Geometry: see drawing. Coordinates: mm, zero at the bounding-box minimum. A direction names the side the tool comes from. Coordinates: 2 decimals unless noted, no trailing zeros. Loops run counter-clockwise (first coordinate to the right, second up) from the corner with the lowest first, then second, coordinate; pieces in that order, holes last. Notation, with made-up numbers: (36.25, -2) -> (76.25, -2) arc R18 cw to (76.25, 10) -> close; hole circle Ø4 at (33.25, 12.5). An arc over 180 degrees is marked (long way). One line per item, written item: value. Start each with the question number.
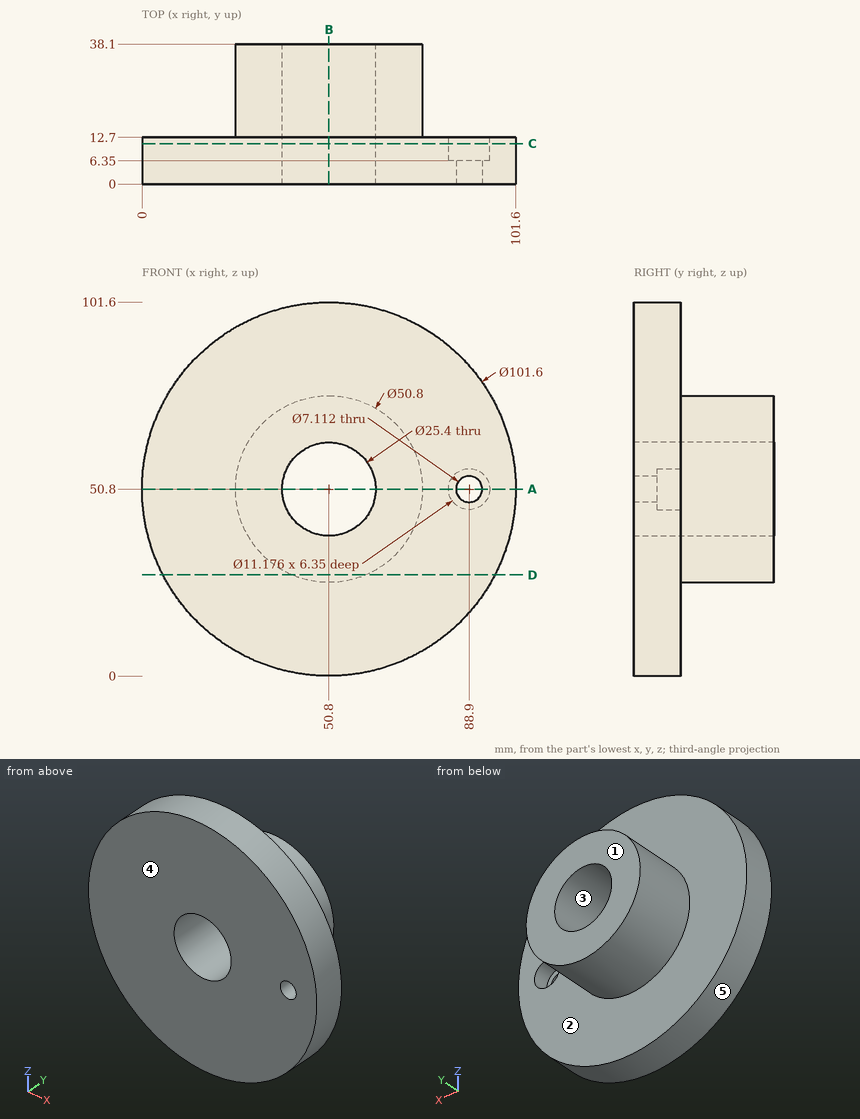
1. Section D-D on z = 27.5. Return the cut outline in (x, y), plus the area to 3 significant figures.
2. Draft query along X for the marked faces 3, 4 and 5. Return one class per face: released by +X, released by -X, zero draft, split by the parting line, or undercut.
3. Section B-B on x = 50.8. Return the cut outline in (y, z).
4. Set-up query: the marked faces 1 and 2. Return all of +Z, -Z, +X, -X, +Y, -Y with unobstructed straight access to the full face (end or side cutting, diameter ignored); none if empty.
5. Section A-A on z = 50.8. Return the cut outline in (x, y).
6. Line query: L1, parallel to X at y = 10.75, z = 50.8; L2, parallel to Z at x = 50, y = 26; L3, parallel to X at y = 19.5, z = 50.8. Output: solid intervals per line, ascending. Write a range as [from, to].
7. Pin query (flat end, axial travel): pin 1 Ø5.5 at (x, z) = (91, 48.5) entering from +Y; pin 2 Ø1.5 at (y, z) = (25, 50) entering from +X; pin 3 Ø5 at (y, z) = (11.5, 21) entering from +X; pin 4 Ø6.5 at (x, z) = (88.9, 50.8) entering from +Y. Return the tip coordinate at first contact, or that it passes through.
8. Section C-C on y = 11. Return the cut outline in (x, z).
Checks:
1. outline: (5.66, 0) -> (95.94, 0) -> (95.94, 12.7) -> (60.91, 12.7) -> (60.91, 38.1) -> (40.69, 38.1) -> (40.69, 12.7) -> (5.66, 12.7) -> close
1. area: 1,660 mm²
2. face 3: undercut
2. face 4: zero draft
2. face 5: split by the parting line
3. outline: (0, 0) -> (12.7, 0) -> (12.7, 25.4) -> (38.1, 25.4) -> (38.1, 38.1) -> (0, 38.1) -> close; (0, 63.5) -> (38.1, 63.5) -> (38.1, 76.2) -> (12.7, 76.2) -> (12.7, 101.6) -> (0, 101.6) -> close
4. face 1: +Z, -Z, +X, -X, +Y
4. face 2: +Y
5. outline: (0, 0) -> (38.1, 0) -> (38.1, 38.1) -> (25.4, 38.1) -> (25.4, 12.7) -> (0, 12.7) -> close; (63.5, 0) -> (85.34, 0) -> (85.34, 6.35) -> (83.31, 6.35) -> (83.31, 12.7) -> (76.2, 12.7) -> (76.2, 38.1) -> (63.5, 38.1) -> close; (92.46, 0) -> (101.6, 0) -> (101.6, 12.7) -> (94.49, 12.7) -> (94.49, 6.35) -> (92.46, 6.35) -> close
6. L1: [0, 38.1], [63.5, 83.31], [94.49, 101.6]
6. L2: [25.41, 38.13], [63.47, 76.19]
6. L3: [25.4, 38.1], [63.5, 76.2]
7. pin 1: y = 12.7
7. pin 2: x = 76.2
7. pin 3: x = 93.64
7. pin 4: through
8. outline: circle Ø101.6 at (50.8, 50.8); hole circle Ø25.4 at (50.8, 50.8); hole circle Ø11.18 at (88.9, 50.8)
